Check sheet for the modelled part. Datum: model origin and axes. Units: mm. Coordinates: 2 decimals unless noted, no trailing zeros. Write each loop counter-clockwise with the first axis right and the second up, starting at its lowest first coordinate (ties: lowest second). Pieces come first, ordered by that corner, then holes. Notation, with made-up numbers: M 55,58.5 L 80,58.5 A20 cw 80,92.5 Z; hole C 38.5,26 d1. An arc over 180 degrees is marked long. Answer as CSV lines item,"result". Start each with the question number.
Q1. Mould release check, pull along X, two halves, no side actions. Record for faces 1 (the cylindrical face through (-5.961, -26.846, 1.479)), 2 (the flat face through (3.9, 20.5, 0)), 3 (the flat face through (0, 0, 2.5)), 4 (the cylindrical face through (19.65, 6.19, 1.23)): pulls with the +X half, pulls with the -X half, needs draft (parallel to the pull), parting line crosses it, or undercut.
Q2. Thickness scan on line 1 along Y through (x, z) = (0, 1.05); line 2 along X through (y, z) = (0.5, 0.3); line 3 along Z through (x, y) = (-4.5, -3). Record the ranges inside material, lowest first. Write a range as from..to.
Q3. Sectioned sample at A-A, the plane x = 0. Record the cut outline in (y, z).
Q4. Depth check by flat-ended pin: pin 1 Ø1.5 at (x, y) = (-21, -20.5) entering from +Z (1 decimal); pin 2 Ø12.5 at (x, y) = (-0.5, -10) entering from -Z. Enter the tip coordinate at first touch or a pass-through.
Q5. Sectioned sample at C-C, the plane z = 1.35. Record the cut outline in (x, y), then the cut area to 3 significant figures.
from build123d import *

# Parameters (mm, degrees)
CYLINDER002_R     = 20.6
CYLINDER002_DEPTH = 2.5
CYLINDER_R        = 27.5
CYLINDER_DEPTH    = 3


with BuildPart() as cylinder002:
    # Cylinder002 → Cylinder002 (new body)
    with BuildSketch(Plane.XY):
        Circle(CYLINDER002_R)
    extrude(amount=CYLINDER002_DEPTH)


with BuildPart() as cone:
    # Cone → Cone (revolve)
    with BuildSketch(Plane(origin=(0, 0, 3), x_dir=(1, 0, 0), z_dir=(0, -1, 0))):
        Polygon((0, 0), (27.5, 0), (22.25, 1.406733), (0, 1.406733), align=None)
    revolve(axis=Axis((0, 0, 3), (0, 0, 1)))


with BuildPart() as obj1:
    # Cylinder → Cylinder (new body)
    with BuildSketch(Plane.XY):
        Circle(CYLINDER_R)
    extrude(amount=CYLINDER_DEPTH)

    # Fusion: union Cone
    add(cone.part)

    # Cut: cut Cylinder002
    add(cylinder002.part, mode=Mode.SUBTRACT)


solid = obj1.part
Output:
1,face 1,"parting line crosses it"
1,face 2,"needs draft"
1,face 3,"undercut"
1,face 4,"undercut"
2,line 1,"y = -27.5..-20.6, 20.6..27.5"
2,line 2,"x = -27.5..-20.59, 20.59..27.5"
2,line 3,"z = 2.5..4.41"
3,outline,"M -27.5,0 L -20.6,0 L -20.6,2.5 L 20.6,2.5 L 20.6,0 L 27.5,0 L 27.5,3 L 22.25,4.41 L -22.25,4.41 L -27.5,3 Z"
4,pin 1,"passes through"
4,pin 2,"stops at z = 2.5"
5,outline,"C 0,0 d55; hole C 0,0 d41.2"
5,area,"1,040 mm^2"
